For this review, take the finished solid that the model builds, in its own axes (mm). A direction names the side the tool comes from. Round coordinates to 2 decimals unless told otherwise and drop trailing zeros. Order: outer loops, then holes, each group sorted by start corner. A loop starts at its lowest first (then second) coordinate and runs counter-clockwise, first axis right, second up. Notation, with made-up numbers: (-38.5, 54.5) - (0.5, 54.5) arc R24 cw to (0.5, 81.5) - close; hole circle Ø3 at (38.5, 6.25). An arc over 180 degrees is marked (long way). One line per question, with ' | ' between items.
Autodesk Inventor part; units mm, degrees
ref_plane "YZ Plane" through (0, 0, 0) normal (1, 0, 0) x (0, 1, 0)
ref_plane "XZ Plane" through (0, 0, 0) normal (0, 1, 0) x (-1, 0, 0)
ref_plane "XY Plane" through (0, 0, 0) normal (0, 0, 1) x (1, 0, 0)
sketch "Sketch1" plane through (0, 0, 0) normal (0, 0, 1) x (1, 0, 0)
  line L0 (0, 0) -> (25.4, 0)
  line L1 (25.4, 0) -> (25.4, 500)
  line L2 (0, 500) -> (25.4, 500)
  line L3 (0, 0) -> (0, 500)
  line L4 (115.4, 0) -> (140.8, 0)
  line L5 (140.8, 0) -> (140.8, 500)
  line L6 (115.4, 500) -> (140.8, 500)
  line L7 (115.4, 0) -> (115.4, 500)
  line L8 (-25, 505) -> (50.4, 505)
  line L9 (50.4, 505) -> (50.4, 429.6)
  line L10 (50.4, 429.6) -> (-25, 429.6)
  line L11 (-25, 429.6) -> (-25, 505)
  circle A0 centre (-17, 437.6) radius 4.5
  circle A1 centre (-17, 497) radius 4.5
  circle A2 centre (42.4, 497) radius 4.5
  circle A3 centre (42.4, 437.6) radius 4.5
  dimension "d0" = 25
  dimension "d31" = 25
  dimension "d32" = 5
  dimension "d33" = 9
  dimension "d34" = 9
  dimension "d35" = 9
  dimension "d36" = 9
  dimension "d37" = 8
  dimension "d38" = 8
  dimension "d39" = 8
  dimension "d40" = 8
  dimension "d41" = 8
  dimension "d42" = 8
  dimension "d43" = 8
  dimension "d44" = 8
extrude "Extrusion1" add sketch "Sketch1" along normal blind 10 contours L10 L11 L8 L9 L1 L2 L3 | L3 L2 L1 L10
sketch "Sketch3" plane through (0, 0, 0) normal (0, 0, -1) x (-1, 0, 0)
  line L0 (5, 505) -> (-30.4, 505)
  line L1 (-30.4, 505) -> (-30.4, 500)
  line L2 (-30.4, 500) -> (5, 500)
  line L3 (5, 500) -> (5, 505)
  line L4 (25, 505) -> (-50.4, 505)
  line L5 (25, 429.6) -> (25, 505)
  point P0 (0, 0)
  dimension "d45" = 35.4
  dimension "d46" = 20
  dimension "d47" = 5
extrude "Extrusion2" add sketch "Sketch3" along normal blind 30.4
sketch "Sketch5" plane through (-5, 500, 0) normal (0, -1, 0) x (1, 0, 0)
  line L0 (0, -30.4) -> (5, -30.4)
  line L1 (5, -30.4) -> (5, 0)
  line L2 (5, 0) -> (0, 0)
  line L3 (0, 0) -> (0, -30.4)
  line L4 (5, -30.4) -> (30.4, -30.4)
  line L5 (30.4, -30.4) -> (30.4, -25.4)
  line L6 (30.4, -25.4) -> (5, -25.4)
  line L7 (5, -25.4) -> (5, -30.4)
  line L8 (35.4, -30.4) -> (30.4, -30.4)
  line L9 (30.4, -30.4) -> (30.4, 0)
  line L10 (30.4, 0) -> (35.4, 0)
  line L11 (35.4, 0) -> (35.4, -30.4)
  line L12 (55.4, 0) -> (-20, 0)
  line L13 (35.4, -30.4) -> (0, -30.4)
  line L14 (0, 0) -> (0, -30.4)
  line L15 (35.4, 0) -> (35.4, -30.4)
  point P0 (5, 0)
  dimension "d48" = 5
  dimension "d49" = 25.4
  dimension "d50" = 25.4
extrude "Extrusion4" add sketch "Sketch5" along normal up to surface (70.4 mm away) contours L3 L2 L1 L0 | L1 L6 L5 L4 | L5 L9 L10 L11 L8
properties part number "CornerBracket" material "PC/ABS Plastic"
(1) We need section A-A on y = 497. State the section outline as (x, z) points, plus the area to 4 significant figures.
Output values:
outline: (-25, 0) - (-21.5, 0) - (-21.5, 10) - (-25, 10) - close; (-12.5, 0) - (-5, 0) - (-5, -30.4) - (30.4, -30.4) - (30.4, 0) - (37.9, 0) - (37.9, 10) - (-12.5, 10) - close; (46.9, 0) - (50.4, 0) - (50.4, 10) - (46.9, 10) - close; hole (0, -25.4) - (25.4, -25.4) - (25.4, 0) - (0, 0) - close | area: 1,005 mm^2
(2) For probe 1 along X at (y, z) = (497, 7); probe 2 along Y at (x, z) = (42.4, 3.75); probe 3 along Z at (x, y) = (10, 469), list the stretches that pass through material, from the lowest coordinate up. Write a range as [from, to].
Output values:
probe 1: [-25, -21.5], [-12.5, 37.9], [46.9, 50.4] | probe 2: [429.6, 433.1], [442.1, 492.5], [501.5, 505] | probe 3: [-30.4, -25.4], [0, 10]
(3) We need section B-B on z = 5. State the section outline as (x, y) points.
Output values:
outline: (-25, 429.6) - (50.4, 429.6) - (50.4, 505) - (-25, 505) - close; hole circle Ø9 at (-17, 437.6); hole circle Ø9 at (-17, 497); hole circle Ø9 at (42.4, 437.6); hole circle Ø9 at (42.4, 497)
(4) Mouldability with a two-part tool opening along Z and no side actions: class faces 4 (the flat face through (0, 465, -13)), 5 (the flat face through (30.4, 468, -15)), 6 (the flat face through (-15, 468, 0)) as released by +Z, released by -Z, zero draft, split by the parting line, or undercut.
Output values:
face 4: undercut | face 5: zero draft | face 6: released by -Z
(5) We need section D-D on x = 42.4. State the section outline as (y, z) points, plus the area to 3 significant figures.
Output values:
outline: (429.6, 0) - (433.1, 0) - (433.1, 10) - (429.6, 10) - close; (442.1, 0) - (492.5, 0) - (492.5, 10) - (442.1, 10) - close; (501.5, 0) - (505, 0) - (505, 10) - (501.5, 10) - close | area: 574 mm^2
(6) We need section C-C on y = 488. State the section outline as (x, z) points.
Output values:
outline: (-25, 0) - (-5, 0) - (-5, -30.4) - (30.4, -30.4) - (30.4, 0) - (50.4, 0) - (50.4, 10) - (-25, 10) - close; hole (0, -25.4) - (25.4, -25.4) - (25.4, 0) - (0, 0) - close
(7) For faces 1 (the flat face through (13, 465, -25.4)), 2 (the flat face through (-5, 467, -15)), 3 (the flat face through (40, 468, 0)), list the 3-axis set-ups (+Z, -Z, +X, -X, +Y, -Y) from which the entire face can be reached by the end or side of a thin tool; tool diameter is ignored.
Output values:
face 1: -Y | face 2: -Z, -X, +Y, -Y | face 3: -Z, +X, +Y, -Y
(8) Insertion check: pin 1 (1.5 mm diameter, centred on x = 39, y = 476, fed in from -Z); pin 2 (1 mm diameter, centred on y = 479.5, z = -23, fed in from -X); pin 3 (4 mm diameter, centred on y = 491.5, z = -17, fed in from +X); pin 4 (8 mm diameter, centred on x = 42.4, y = 437.6, fed in from -Z). Each pin has a flat end and moves straight along its axis. Give the tip position at first contact, or say it passes through.
Output values:
pin 1: z = 0 | pin 2: x = -5 | pin 3: x = 30.4 | pin 4: through
